Input: part model. Units: mm. Frame: model coordinates. Face numbers are marked on the shaded views. A direction names the side the tool comes from. Coordinates: 2 decimals unless noted, no trailing zeros. Order: outer loops, then holes, each group sorted by start corner. A loop starts at its lowest first (then second) coordinate and runs counter-clockwise, first axis right, second up. Notation, with made-up numbers: (56.25, 71.25) -> (114.25, 71.25) arc R13 ccw to (114.25, 91.25) -> close; hole circle Ø1 at (54.25, 19.5). An arc over 180 degrees is marked (long way). Write each question's results on one line, items separated by ' | '.
```python
from build123d import *

# Parameters (mm, degrees)
SKETCH_W        = 46
SKETCH_H        = 28
PAD_DEPTH       = 46
SKETCH001_W     = 46
SKETCH001_H     = 46
POCKET_DEPTH    = 9.333333
FILLET_R        = 2.5
SKETCH002_R     = 20
POCKET001_DEPTH = 2.5
SKETCH003_R     = 15
POCKET002_DEPTH = 2.5
SKETCH004_R     = 7.5
PAD001_DEPTH    = 1
FILLET001_R     = 1.5
FILLET002_R     = 0.75


with BuildPart() as part:
    # Sketch → Pad (new body)
    with BuildSketch(Plane.XY):
        Rectangle(SKETCH_W, SKETCH_H)
    extrude(amount=PAD_DEPTH)

    # Sketch001 (on Face4 of Pad) → Pocket (cut)
    with BuildSketch(Plane(origin=(0, 14, 0), x_dir=(-1, 0, 0), z_dir=(0, 1, 0))):
        with Locations((0, 23)):
            Rectangle(SKETCH001_W, SKETCH001_H)
        with BuildLine():
            Line((-22, 40), (-22, 6))
            ThreePointArc((-17, 1), (-18.464466, 4.535534), (-22, 6))
            Line((-17, 1), (17, 1))
            ThreePointArc((22, 6), (18.464466, 4.535534), (17, 1))
            Line((22, 6), (22, 40))
            ThreePointArc((17, 45), (18.464466, 41.464466), (22, 40))
            Line((17, 45), (-17, 45))
            ThreePointArc((-22, 40), (-18.464466, 41.464466), (-17, 45))
        make_face(mode=Mode.SUBTRACT)
    extrude(amount=-POCKET_DEPTH, mode=Mode.SUBTRACT)

    # Fillet
    fillet_edges = [part.edges().sort_by_distance(p)[0] for p in [
        (23, -4.666666, 46),
        (-23, -4.666666, 46),
        (-23, -4.666666, 0),
        (23, -4.666666, 0),
        (-22, 9.333334, 6),
        (-17, 9.333334, 1),
        (17, 9.333334, 1),
        (22, 9.333334, 6),
        (22, 9.333334, 40),
        (17, 9.333334, 45),
        (-17, 9.333334, 45),
        (-22, 9.333334, 40),
    ]]
    fillet(fillet_edges, radius=FILLET_R)

    # Sketch002 (on Face2 of Fillet) → Pocket001 (cut)
    with BuildSketch(Plane.XZ.offset(14)):
        with Locations((0, 23.846073)):
            Circle(SKETCH002_R)
    extrude(amount=-POCKET001_DEPTH, mode=Mode.SUBTRACT)

    # Sketch003 (on Face28 of Pocket001) → Pocket002 (cut)
    with BuildSketch(Plane.XZ.offset(11.5)):
        with Locations((0, 23.846073)):
            Circle(SKETCH003_R)
    extrude(amount=-POCKET002_DEPTH, mode=Mode.SUBTRACT)

    # Sketch004 (on Face31 of Pocket002) → Pad001 (join)
    with BuildSketch(Plane.XZ.offset(9)):
        with Locations((0, 23.846073)):
            Circle(SKETCH004_R)
    extrude(amount=PAD001_DEPTH)

    # Fillet001
    fillet001_edges = [part.edges().sort_by_distance(p)[0] for p in [
        (-15, -11.5, 23.846073),
    ]]
    fillet(fillet001_edges, radius=FILLET001_R)

    # Fillet002
    fillet002_edges = [part.edges().sort_by_distance(p)[0] for p in [
        (-7.5, -10, 23.846073),
    ]]
    fillet(fillet002_edges, radius=FILLET002_R)


solid = part.part
```
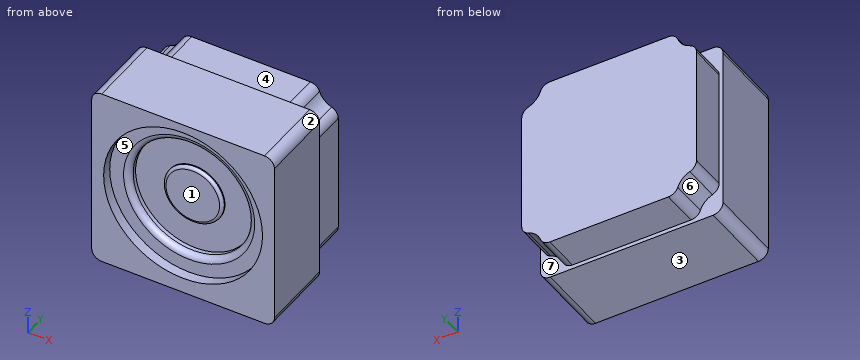
(1) Pin query (flat end, axial travel): P1, Ø10.5, axis at y = 11, z = 17.5, coming from the -X side; P2, Ø24, axis at x = 0, z = 23.85, coming from the -Y side; P3, Ø10.5, axis at y = 10, z = 25, coming from the +X side; P4, Ø24, axis at x = 5.5, z = 17.5, coming from the -Y side. Return the tip coordinate at first contact, or that it passes through.
Return value:
P1: x = -22 | P2: y = -10 | P3: x = 22 | P4: y = -14
(2) Cut plane B-B, the plane z = 41. Return loops of the section in (x, y), plus the area to 3 significant figures.
Return value:
outline: (-23, -14) -> (-10.28, -14) -> (-10.28, -11.5) -> (10.28, -11.5) -> (10.28, -14) -> (23, -14) -> (23, 4.67) -> (19, 4.67) -> (19, 14) -> (-19, 14) -> (-19, 4.67) -> (-23, 4.67) -> close | area: 1,160 mm2
(3) Line query: line 1 along Z through (x, y) = (0, -13.2); line 2 along Z through (x, y) = (0, -9.35); line 3 along Z through (x, y) = (5, -9.5). Output: solid intervals per line, ascending. Write a range as from..to.
Return value:
line 1: 0..3.85, 43.85..46 | line 2: 0..8.85, 16.35..31.34, 38.85..46 | line 3: 0..9.7, 18.31..29.38, 37.99..46
(4) Mould query, pull axis X, two halves, no side actions, for the marked faces 1, 2 and 3. Classes: +X half, -X half, draft (parallel to the pull), parting line (faces both ways), or undercut.
Return value:
face 1: undercut | face 2: +X half | face 3: draft
(5) Reachability of the marked faces 4, 5, 6 and 7 from +Z, -Z, +X, -X, +Y, -Y: full face, straight path, thin tool, end or side. Return the list, or none.
Return value:
face 4: +Z, +X, -X, +Y | face 5: -Y | face 6: -Z, -X, +Y | face 7: +Y
(6) Cut plane C-C, the plane x = 18. Return loops of the section in (y, z).
Return value:
outline: (-14, 0) -> (4.67, 0) -> (4.67, 4) -> (14, 4) -> (14, 42) -> (4.67, 42) -> (4.67, 46) -> (-14, 46) -> (-14, 32.56) -> (-11.5, 32.56) -> (-11.5, 15.13) -> (-14, 15.13) -> close
(7) Cut plane A-A, the plane x = 0. Return loops of the section in (y, z).
Return value:
outline: (-14, 0) -> (4.67, 0) -> (4.67, 1) -> (14, 1) -> (14, 45) -> (4.67, 45) -> (4.67, 46) -> (-14, 46) -> (-14, 43.85) -> (-11.5, 43.85) -> (-11.5, 40.35) arc R1.5 ccw to (-10, 38.85) -> (-9, 38.85) -> (-9, 31.35) -> (-9.25, 31.35) arc R0.75 ccw to (-10, 30.6) -> (-10, 17.1) arc R0.75 ccw to (-9.25, 16.35) -> (-9, 16.35) -> (-9, 8.85) -> (-10, 8.85) arc R1.5 ccw to (-11.5, 7.35) -> (-11.5, 3.85) -> (-14, 3.85) -> close
